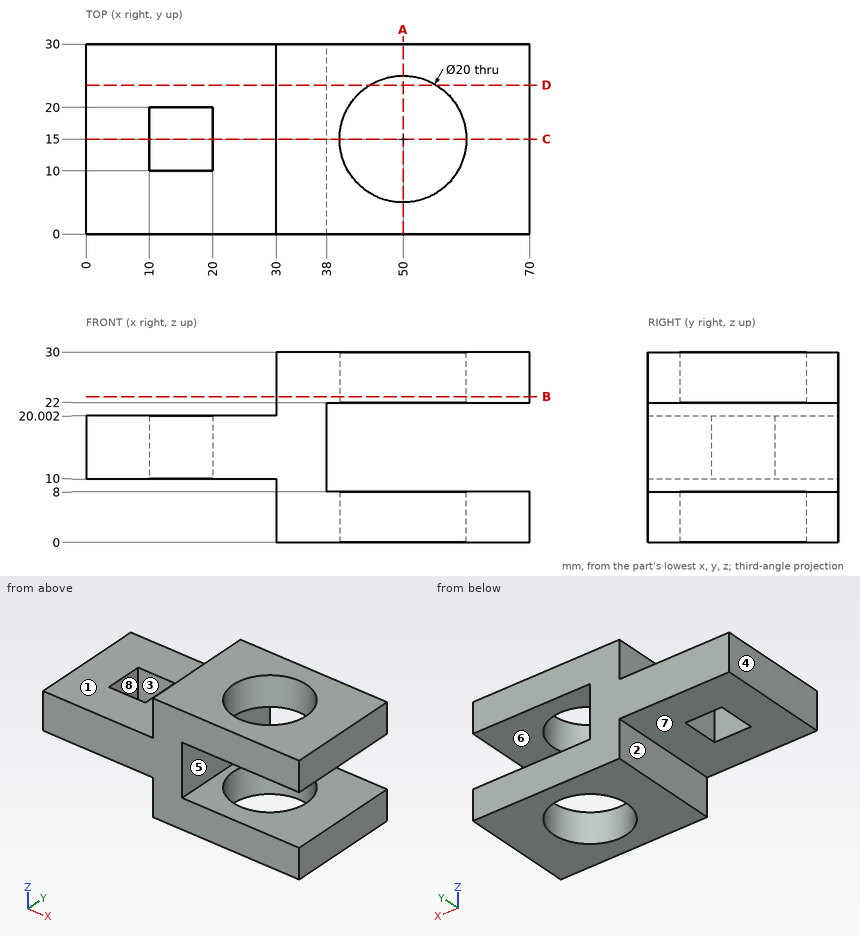
For this review, use the dimensioned drawing (mm, ordinates from the lowest corner) and the shaded views. A direction names the side the tool comes from. Coordinates: 2 decimals unless noted, no trailing zeros. Write each loop counter-clockwise with the first axis right and the second up, starting at its lowest first coordinate (ties: lowest second). Pieces come first, ordered by that corner, then holes. Notation, with made-up numbers: (17, 13.5) - (44, 13.5) arc R34 ccw to (44, 44.5) - close; hole circle Ø7 at (86, -13.75). An arc over 180 degrees is marked (long way). Answer as a JSON object with one key per item and string values. Group by question number.
1. Add section B-B (z = 23). Give the boundary of the cut face in (x, y).
2. Machinability: for the marked faces 1, 2, 3, 4 and 5, which of the approach directions +Z, -Z, +X, -X, +Y, -Y give a long, thin tool a straight path to every point of the face, cutting with its end or side? Answer none if there is none.
3. Add section C-C (y = 15). Give the boundary of the cut face in (x, z).
4. Mouldability with a two-part tool opening along Z and no side actions: class the marked faces 6, 7 and 8 as pulls with the +Z half, pulls with the -Z half, needs draft (parallel to the pull), parting line crosses it, or undercut.
5. Add section A-A (x = 50). Give the boundary of the cut face in (y, z).
6. Add section D-D (y = 23.5). Give the boundary of the cut face in (x, z).
7. Clearance check with flat-ended pins moving along their axes: pin 1 Ø2 at (x, y) = (10.5, 21) entering from +Z; pin 2 Ø3 at (y, z) = (15, 4) entering from -X; pin 3 Ø8 at (y, z) = (16.5, 12.5) entering from +X. State where each tip first meets the part, or that it passes through.
8. To check wall thickness, follow probe 1 along X at (y, z) = (15, 3); probe 2 along Z at (x, y) = (38.5, 8.25); probe 3 along Y at (x, z) = (50, 5). State the ranges of each line that lie inside material, in increasing order.
Findings:
{
 "1": {"outline": "(30, 0) - (70, 0) - (70, 30) - (30, 30) - close; hole circle Ø20 at (50, 15)"},
 "2": {"face 1": "+Z, -X, +Y, -Y", "face 2": "-Z, -X, +Y, -Y", "face 3": "+Z, -Z", "face 4": "+Z, -Z, -X, +Y, -Y", "face 5": "+X, +Y, -Y"},
 "3": {"outline": "(0, 10) - (10, 10) - (10, 20) - (0, 20) - close; (20, 10) - (30, 10) - (30, 0) - (40, 0) - (40, 8) - (38, 8) - (38, 22) - (40, 22) - (40, 30) - (30, 30) - (30, 20) - (20, 20) - close; (60, 0) - (70, 0) - (70, 8) - (60, 8) - close; (60, 22) - (70, 22) - (70, 30) - (60, 30) - close"},
 "4": {"face 6": "undercut", "face 7": "pulls with the -Z half", "face 8": "needs draft"},
 "5": {"outline": "(0, 0) - (5, 0) - (5, 8) - (0, 8) - close; (0, 22) - (5, 22) - (5, 30) - (0, 30) - close; (25, 0) - (30, 0) - (30, 8) - (25, 8) - close; (25, 22) - (30, 22) - (30, 30) - (25, 30) - close"},
 "6": {"outline": "(0, 10) - (30, 10) - (30, 0) - (44.73, 0) - (44.73, 8) - (38, 8) - (38, 22) - (44.73, 22) - (44.73, 30) - (30, 30) - (30, 20) - (0, 20) - close; (55.27, 0) - (70, 0) - (70, 8) - (55.27, 8) - close; (55.27, 22) - (70, 22) - (70, 30) - (55.27, 30) - close"},
 "7": {"pin 1": "z = 20", "pin 2": "x = 30", "pin 3": "x = 38"},
 "8": {"probe 1": "30 to 40, 60 to 70", "probe 2": "0 to 8, 22 to 30", "probe 3": "0 to 5, 25 to 30"}
}
